The drawing under review shows one solid part. Ordinate dimensions are in mm from its lowest x, y, z. A direction names the side the tool comes from. Coordinates: 2 decimals unless noted, no trailing zeros. Write each loop counter-clockwise with the first axis right and the second up, starting at its lowest first coordinate (ties: lowest second). Pieces come first, ordered by that corner, then holes. Notation, with made-up numbers: (68.25, 11.25) - (77.25, 11.25) arc R26 cw to (77.25, 40.25) - close; hole circle Ø6 at (-5.75, -35.5). An arc over 180 degrees is marked (long way). Put each result on its own line as item: value. Start each with the question number.
Item 1: Consider section B-B on x = 8. Give the boundary of the cut face in (y, z).
Item 2: Consider section D-D on y = 24. Give the boundary of the cut face in (x, z).
Item 3: For pin 1 (1.5 mm diameter, centred on x = 36.5, z = 9.5, fed in from +Y); pin 2 (13.5 mm diameter, centred on x = 30, y = 21, fed in from +Z); pin 3 (1.7 mm diameter, centred on y = 6.5, z = 6, fed in from -X), all flat-tipped, find the tip position at first contact; note any pin that passes through.
Item 4: Consider section C-C on z = 2.75. Give the boundary of the cut face in (x, y), then the cut area to 3 significant figures.
Item 5: Consider section A-A on z = 10. Give the boundary of the cut face in (x, y).
Item 6: Machinability: for the marked faces 1, 2 and 3, which of the approach directions +Z, -Z, +X, -X, +Y, -Y give a long, thin tool a straight path to every point of the face, cutting with its end or side? Answer none if there is none.
Item 7: Mouldability with a two-part tool opening along Y and no side actions: class the marked faces 4, 5, 6 and 7 as pulls with the +Y half, pulls with the -Y half, needs draft (parallel to the pull), parting line crosses it, or undercut.
Item 8: To check wall thickness, follow L1, parallel to X at y = 3.5, z = 10; L2, parallel to Y at x = 30, z = 3.5; L3, parallel to Y at x = 30.5, z = 17. State the ranges of each line that lie inside material, in increasing order. Write a range as [from, to].
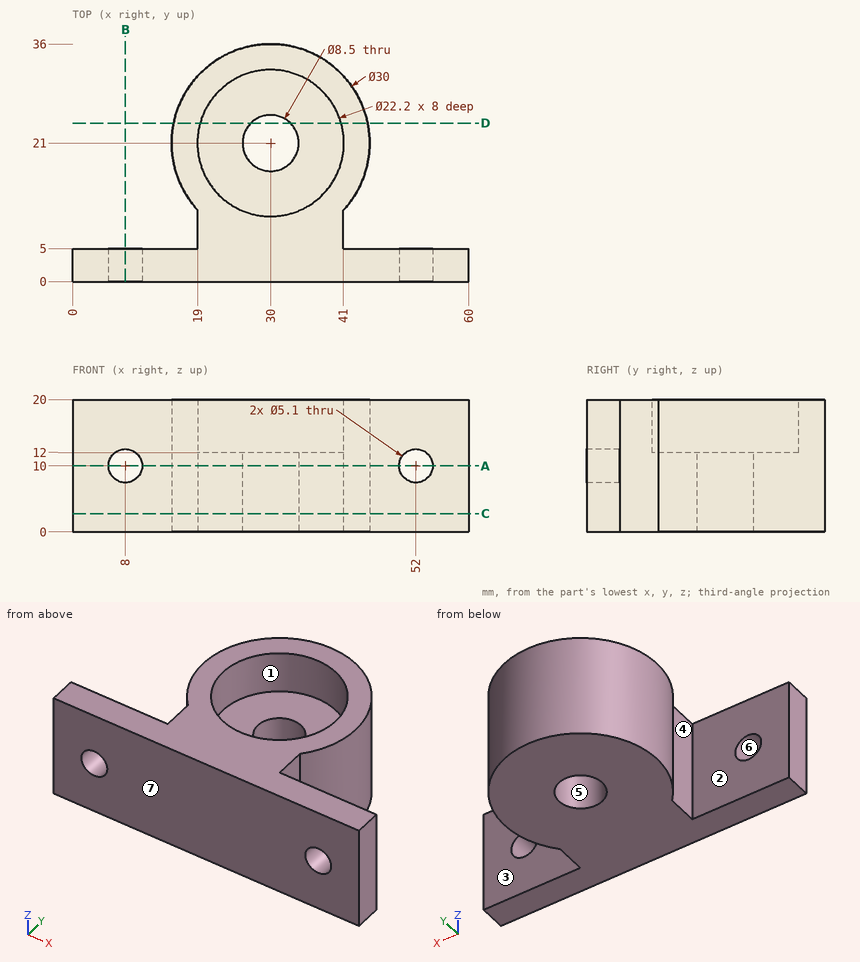
Report:
1. outline: (0, 0) - (5, 0) - (5, 7.45) - (0, 7.45) - close; (0, 12.55) - (5, 12.55) - (5, 20) - (0, 20) - close
2. outline: (15.3, 0) - (26.99, 0) - (26.99, 12) - (19.31, 12) - (19.31, 20) - (15.3, 20) - close; (33.01, 0) - (44.7, 0) - (44.7, 20) - (40.69, 20) - (40.69, 12) - (33.01, 12) - close
3. pin 1: y = 34.85
3. pin 2: z = 12
3. pin 3: x = 19
4. outline: (0, 0) - (60, 0) - (60, 5) - (41, 5) - (41, 10.8) arc R15 ccw (long way) to (19, 10.8) - (19, 5) - (0, 5) - close; hole circle Ø8.5 at (30, 21)
4. area: 1,000 mm²
5. outline: (0, 0) - (5.45, 0) - (5.45, 5) - (0, 5) - close; (10.55, 0) - (49.45, 0) - (49.45, 5) - (41, 5) - (41, 10.8) arc R15 ccw (long way) to (19, 10.8) - (19, 5) - (10.55, 5) - close; (54.55, 0) - (60, 0) - (60, 5) - (54.55, 5) - close; hole circle Ø8.5 at (30, 21)
6. face 1: +Z
6. face 2: +Z, -Z, -X
6. face 3: +Z, -Z, +X
7. face 4: undercut
7. face 5: undercut
7. face 6: needs draft
7. face 7: pulls with the -Y half
8. L1: [0, 5.45], [10.55, 49.45], [54.55, 60]
8. L2: [0, 16.75], [25.25, 36]
8. L3: [0, 9.91], [32.09, 35.99]
